For this review, use the dimensioned drawing (mm, ordinates from the lowest corner) and the shaded views. Give positions to 0.01 mm unless a question says otherwise; leave off trailing zeros. Order: outer loops, then holes, each group sorted by start corner. A loop starts at its lowest first (then second) coordinate and runs counter-clockwise, first axis right, second up. Notation, with made-up numbers: (-12.75, 29.5) - (-8.75, 29.5) arc R25 cw to (-8.75, 55.5) - close; hole circle Ø10 at (31, -13.75). An arc over 180 degrees is marked (long way). Use a Markdown table: item, result. Add a question column.
1) We need section C-C on z = 3.15. Give the number of separate pieces and of enclosed holes in the cut face, then the cut area to 3 significant figures.
2) We need section A-A on y = 84. Write out the cut boundary in (x, z), then the cut area to 3 significant figures.
3) We need section B-B on x = 26. Write out the cut boundary in (y, z), then the cut area to 3 significant figures.
4) Clearance check with a flat-ended pin moving along its axis: P1, Ø2, axis at x = 55, y = 84, coming from the +Z side. State where the tip first meets the part, or that it passes through.
5) Wall thickness on L1, parallel to X at y = 123.5, z = 1.7; L2, parallel to X at y = 56, z = 2.6; L3, parallel to Y at x = 59.5, z = 4.2: over which ranges is each line inside the solid? List them lowest first.
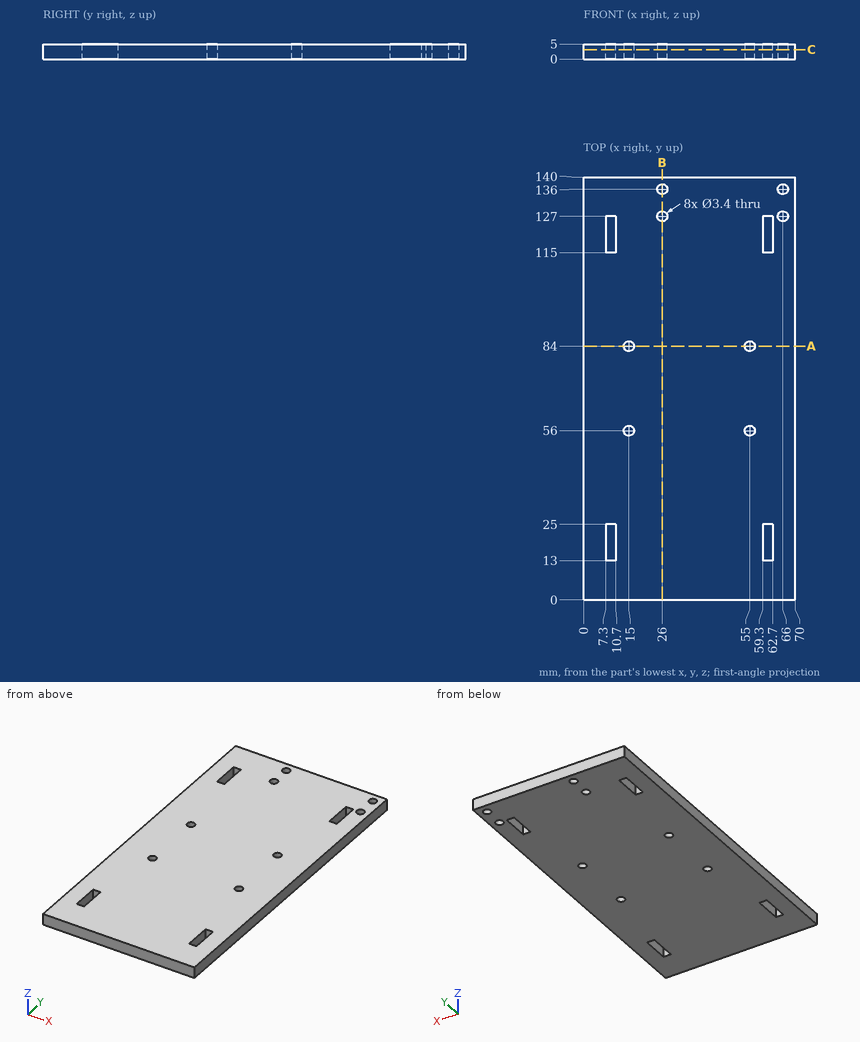
Checked values:
| question | item | result |
|---|---|---|
| 1 | separate pieces | 1 |
| 1 | enclosed holes | 12 |
| 1 | area | 9,560 mm² |
| 2 | outline | (0, 0) - (13.3, 0) - (13.3, 5) - (0, 5) - close; (16.7, 0) - (53.3, 0) - (53.3, 5) - (16.7, 5) - close; (56.7, 0) - (70, 0) - (70, 5) - (56.7, 5) - close |
| 2 | area | 316 mm² |
| 3 | outline | (0, 0) - (125.3, 0) - (125.3, 5) - (0, 5) - close; (128.7, 0) - (134.3, 0) - (134.3, 5) - (128.7, 5) - close; (137.7, 0) - (140, 0) - (140, 5) - (137.7, 5) - close |
| 3 | area | 666 mm² |
| 4 | P1 | through |
| 5 | L1 | 0 to 7.3, 10.7 to 59.3, 62.7 to 70 |
| 5 | L2 | 0 to 13.3, 16.7 to 53.3, 56.7 to 70 |
| 5 | L3 | 0 to 13, 25 to 115, 127 to 140 |
